Answer from the drawing. Dimensions are ordinates in mm from the lowest x, y and z of the part. A direction names the side the tool comes from. Round coordinates to 2 decimals unless told otherwise and drop trailing zeros. Order: outer loops, then holes, each group sorted by start corner. A loop starts at its lowest first (then second) coordinate and runs counter-clockwise, first axis right, second up.
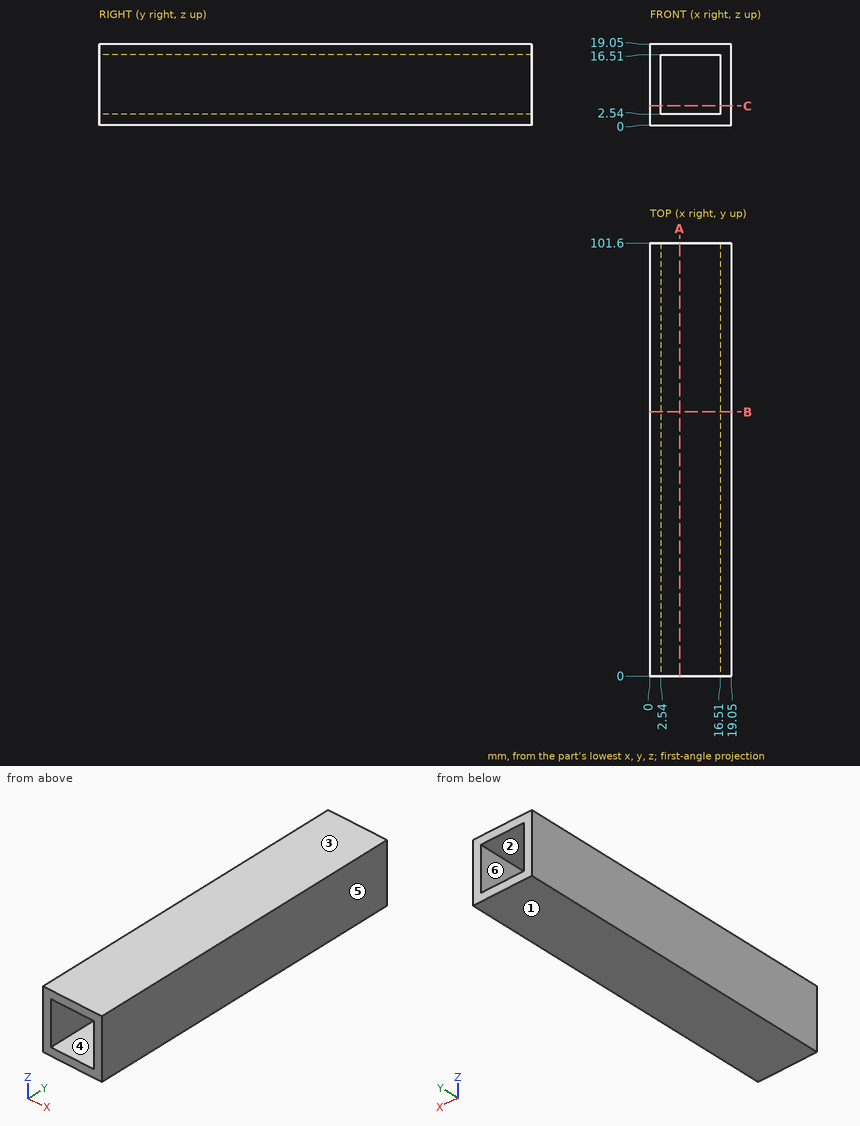
Q1. A cutting plane is placed at A-A, the plane x = 7. Give the vertices of the cut face in (y, z).
Outcome:
outline: (0, 0) - (101.6, 0) - (101.6, 2.54) - (0, 2.54) - close; (0, 16.51) - (101.6, 16.51) - (101.6, 19.05) - (0, 19.05) - close
Q2. A flat-ended cylindrical pin translates along its axis: pin 1 (1 mm diameter, centred on x = 15, z = 8, fed in from +Y). Find the tip coordinate at first contact, or state that the pin passes through.
Outcome:
pin 1: passes through
Q3. For a pull along Z with two mould halves and no side action, classify the marked faces 3, 4, 5 and 6 as released by +Z, released by -Z, zero draft, split by the parting line, or undercut.
Outcome:
face 3: released by +Z
face 4: undercut
face 5: zero draft
face 6: undercut
Q4. A cutting plane is placed at B-B, the plane y = 62. Give the vertices of the cut face in (x, z).
Outcome:
outline: (0, 0) - (19.05, 0) - (19.05, 19.05) - (0, 19.05) - close; hole (2.54, 2.54) - (16.51, 2.54) - (16.51, 16.51) - (2.54, 16.51) - close
Q5. For the marked faces 1 and 2, determine the directions among +Z, -Z, +X, -X, +Y, -Y from which every point of the face is accessible in a straight line to the end or side of a thin tool.
Outcome:
face 1: -Z, +X, -X, +Y, -Y
face 2: +Y, -Y
Q6. A cutting plane is placed at C-C, the plane z = 4.5. Give the vertices of the cut face in (x, y), plus the area to 3 significant figures.
Outcome:
outline: (0, 0) - (2.54, 0) - (2.54, 101.6) - (0, 101.6) - close; (16.51, 0) - (19.05, 0) - (19.05, 101.6) - (16.51, 101.6) - close
area: 516 mm2
Q7. A straight line is drawn through the part: probe 1 along X at (y, z) = (8.5, 13.75). Find the intervals that lie inside material, in ascending order.
Outcome:
probe 1: x = 0 to 2.54, 16.51 to 19.05
